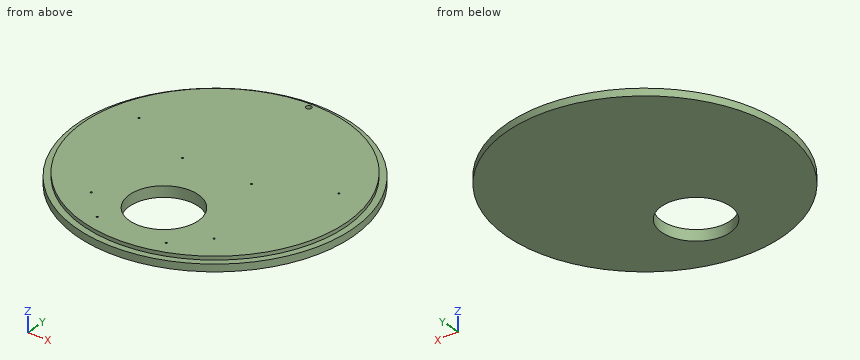
```python
from build123d import *

# Parameters (mm, degrees)
SKETCH058_R     = 152.5
PAD_DEPTH       = 8
SKETCH059_R     = 145.5
PAD017_DEPTH    = 4
SKETCH003_R     = 38
POCKET_DEPTH    = 12.001
SKETCH054_R     = 3
SKETCH054_R_2   = 1
POCKET019_DEPTH = 6


with BuildPart() as part:
    # Sketch058 → Pad (new body)
    with BuildSketch(Plane.XY):
        Circle(SKETCH058_R)
    extrude(amount=PAD_DEPTH)

    # Sketch059 (on DatumPlane) → Pad017 (join)
    with BuildSketch(Plane.XY.offset(8)):
        Circle(SKETCH059_R)
    extrude(amount=PAD017_DEPTH)

    # Sketch003 → Pocket (cut, through all)
    with BuildSketch(Plane.XY):
        with Locations((0, -76.25)):
            Circle(SKETCH003_R)
    extrude(amount=POCKET_DEPTH, mode=Mode.SUBTRACT)

    # Sketch054 → Pocket019 (cut)
    with BuildSketch(Plane.XY.offset(12)):
        with Locations((0, 140)):
            Circle(SKETCH054_R)
        with Locations((109.993235, 35.738968)):
            Circle(SKETCH054_R_2)
        with Locations((67.651258, -93.113968)):
            Circle(SKETCH054_R_2)
        with Locations((-67.651258, -93.113968)):
            Circle(SKETCH054_R_2)
        with Locations((-109.993235, 35.738968)):
            Circle(SKETCH054_R_2)
        with Locations((-38, 2.75)):
            Circle(SKETCH054_R_2)
        with Locations((38, 2.75)):
            Circle(SKETCH054_R_2)
        with Locations((-38, -124.25)):
            Circle(SKETCH054_R_2)
        with Locations((38, -124.25)):
            Circle(SKETCH054_R_2)
    extrude(amount=-POCKET019_DEPTH, mode=Mode.SUBTRACT)


with BuildPart() as part_1:
    # Body placement: moved
    add(part.part.moved(Location((444.217634, -154.760103, 0))))


solid = part_1.part
```
Here's how the part is built. I have some questions about the finished solid (model axes, mm). Coordinates: 2 decimals unless noted, no trailing zeros. Order: outer loops, then holes, each group sorted by start corner. A loop starts at its lowest first (then second) coordinate and runs counter-clockwise, first axis right, second up.
1) Will these pins go through, and if not, where does the flat tip stop? pin 1 (1.2 mm diameter, centred on x = 554.21, y = -119.02, fed in from +Z); pin 2 (2 mm diameter, centred on x = 510.5, z = 4.5, fed in from -Y); pin 3 (1.5 mm diameter, centred on y = -219.5, z = 6, fed in from +X).
2) Imagine slicing it at D-D on y = -101. List the corners of the cut face in (x, z) for me.
3) I need wall thicknesses on line 1 (Y direction, x = 462, z = 7); line 2 (Y direction, x = 453, z = 2.25); line 3 (X direction, y = -204, z = 8.75). Which ranges of each line are inside material? Lowest first, please.
4) Imagine slicing it at B-B on y = -199. List the corners of the cut face in (x, z) for me.
5) Imagine slicing it at C-C on x = 562. List the corners of the cut face in (y, z) for me.
6) Imagine slicing it at A-A on x = 462. List the corners of the cut face in (y, z) for me, and give its area (3 significant figures).
Response values:
1. pin 1: stops at z = 6
1. pin 2: stops at y = -292.58
1. pin 3: stops at x = 582.64
2. outline: (301.51, 0) - (586.93, 0) - (586.93, 8) - (579.42, 8) - (579.42, 12) - (309.01, 12) - (309.01, 8) - (301.51, 8) - close
3. line 1: y = -306.22 to -264.59, -197.43 to -3.3
3. line 2: y = -307.01 to -267.98, -194.04 to -2.51
3. line 3: x = 307.3 to 417.49, 470.95 to 581.13
4. outline: (298.28, 0) - (423.74, 0) - (423.74, 12) - (305.61, 12) - (305.61, 8) - (298.28, 8) - close; (464.7, 0) - (590.16, 0) - (590.16, 8) - (582.83, 8) - (582.83, 12) - (464.7, 12) - close
5. outline: (-251.63, 0) - (-57.89, 0) - (-57.89, 8) - (-69.33, 8) - (-69.33, 12) - (-240.19, 12) - (-240.19, 8) - (-251.63, 8) - close
6. outline: (-306.22, 0) - (-264.59, 0) - (-264.59, 12) - (-299.17, 12) - (-299.17, 8) - (-306.22, 8) - close; (-197.43, 0) - (-3.3, 0) - (-3.3, 8) - (-10.35, 8) - (-10.35, 12) - (-197.43, 12) - close
6. area: 2,770 mm2
